Build history of the part. All positions in model axes, mm. A direction names the side the tool comes from. Round coordinates to 2 decimals unless told otherwise and drop trailing zeros. Write each loop counter-clockwise with the first axis right and the second up, starting at its lowest first coordinate (ties: lowest second). Pieces come first, ordered by that corner, then holes. Notation, with made-up numbers: M 52.25,-2 L 91.25,-2 A29 cw 91.25,21 Z; hole C -25.75,45 d5. An arc over 180 degrees is marked long. One line per item, written item: value. Start each with the question number.
```python
from build123d import *

# Parameters (mm, degrees)
SKETCH1_R               = 40
SKETCH1_R_2             = 7.5
BOSS_EXTRUDE1_DEPTH     = 7.5
CUT_EXTRUDE1_REACH      = 59.064
CUT_EXTRUDE1_END_RADIUS = 40
SKETCH2_R               = 2
CUT_EXTRUDE2_REACH      = 99.064
CUT_EXTRUDE2_END_RADIUS = 7.5
CUT_EXTRUDE2_START      = 40
SKETCH2_2_R             = 2


with BuildPart() as part:
    # Sketch1 → Boss-Extrude1 (new, symmetric)
    with BuildSketch(Plane.XY):
        Circle(SKETCH1_R)
        with Locations((26, 0)):
            Circle(SKETCH1_R_2, mode=Mode.SUBTRACT)
        with BuildLine():
            Line((4.769696007, 1.5), (6.5, 1.5))
            Line((6.5, 1.5), (6.5, -1.5))
            Line((6.5, -1.5), (4.769696007, -1.5))
            ThreePointArc((4.769696007, -1.5), (-5, 0), (4.769696007, 1.5))
        make_face(mode=Mode.SUBTRACT)
    extrude(amount=BOSS_EXTRUDE1_DEPTH, both=True)

    # Cut-Extrude1: up to this cylinder (the profile starts inside it)
    cut_extrude1_end = Plane(origin=(0, 0, 0), z_dir=(0, 0, -1)) * Cylinder(CUT_EXTRUDE1_END_RADIUS, 199.128, mode=Mode.PRIVATE)
    # Sketch2 → Cut-Extrude1 (cut, up to the surface)
    with BuildSketch(Plane(origin=(0, 0, 0), x_dir=(0, 0, -1), z_dir=(1, 0, 0)), mode=Mode.PRIVATE) as cut_extrude1_sk1:
        Circle(SKETCH2_R)
    cut_extrude1_tool1 = extrude(cut_extrude1_sk1.sketch, amount=-CUT_EXTRUDE1_REACH, mode=Mode.PRIVATE) & cut_extrude1_end
    add(cut_extrude1_tool1.solids().sort_by_distance((0, 0, 0))[0], mode=Mode.SUBTRACT)

    # Cut-Extrude2: up to this cylinder (the profile starts outside it)
    cut_extrude2_end = Plane(origin=(26, 0, 0), z_dir=(0, 0, -1)) * Cylinder(CUT_EXTRUDE2_END_RADIUS, 214.128, mode=Mode.PRIVATE)
    # Sketch2<2> → Cut-Extrude2 (cut, up to the surface)
    with BuildSketch(Plane(origin=(0, 0, 0), x_dir=(0, 0, -1), z_dir=(1, 0, 0)).offset(CUT_EXTRUDE2_START), mode=Mode.PRIVATE) as cut_extrude2_sk1:
        Circle(SKETCH2_2_R)
    cut_extrude2_tool1 = extrude(cut_extrude2_sk1.sketch, amount=-CUT_EXTRUDE2_REACH, mode=Mode.PRIVATE) - cut_extrude2_end
    add(cut_extrude2_tool1.solids().sort_by_distance((40, 0, 0))[0], mode=Mode.SUBTRACT)


solid = part.part
```
Item 1: Which spindle directions (+Z, -Z, +X, -X, +Y, -Y) get a long thin tool onto all of the face, cutting with end or side? Do faces 1 (the flat face through (-1, -8, 7.5)), 2 (the flat face through (6.5, 0, 0)), 3 (the cylindrical face through (37, -2, 0)). Say none if no direction does.
Item 2: Two-plate mould, pull along X, no slides. Class faces 4 (the cylindrical face through (-22, -2, 0)), 5 (the flat face through (6, -1.5, 0)), 6 (the cylindrical face through (38.153, 12.015, 0.105)), 7 (the cylindrical face through (18.507, 0.33, -0.105)): pulls with the +X half, pulls with the -X half, needs draft (parallel to the pull), parting line crosses it, or undercut.
Item 3: Cut at D-D, the plane z = 0. Write the cut outline in (x, y).
Item 4: Cut at C-C, the plane z = -5. Write the cut outline in (x, y).
Item 5: Drill centre lines: line 1 (Y direction, x = 0, z = 3); line 2 (Z direction, x = 38.5, y = 0); line 3 (Y direction, x = -34, z = 1.25). Where is each one in solid material? Low to high.
Item 6: Cut at B-B, the plane y = 0. Write the cut outline in (x, z), plus the area to 4 significant figures.
Item 7: Drop flat-ended pins along their axis: pin 1 (5 mm diameter, centred on y = -20.5, z = -1, fed in from -X); pin 2 (3 mm diameter, centred on x = 8.5, z = 5.5, fed in from +Y); pin 3 (3 mm diameter, centred on y = 0, z = 0, fed in from +X); pin 4 (24 mm diameter, centred on x = 26, y = 0, fed in from -Z). Give the stop position or say it passes through.
Item 8: Cut at A-A, the plane x = 0. Write the cut outline in (y, z), plus the area to 3 significant figures.
Computed values:
1. face 1: +Z, +X, -X, +Y, -Y
1. face 2: +Z, -Z
1. face 3: +X
2. face 4: needs draft
2. face 5: undercut
2. face 6: parting line crosses it
2. face 7: undercut
3. outline: M -39.95,-2 A40 ccw 39.95,-2 L 33.23,-2 A7.5 cw long 33.23,2 L 39.95,2 A40 ccw -39.95,2 L -4.58,2 A5 cw 4.77,1.5 L 6.5,1.5 L 6.5,-1.5 L 4.77,-1.5 A5 cw -4.58,-2 Z
4. outline: C 0,0 d80; hole M 4.77,-1.5 L 6.5,-1.5 L 6.5,1.5 L 4.77,1.5 A5 ccw long Z; hole C 26,0 d15
5. line 1: y = -40 to -5, 5 to 40
5. line 2: z = -7.5 to -2, 2 to 7.5
5. line 3: y = -21.07 to -1.56, 1.56 to 21.07
6. outline: M -40,-7.5 L -5,-7.5 L -5,-2 L -40,-2 Z; M -40,2 L -5,2 L -5,7.5 L -40,7.5 Z; M 6.5,-7.5 L 18.5,-7.5 L 18.5,7.5 L 6.5,7.5 Z; M 33.5,-7.5 L 40,-7.5 L 40,-2 L 33.5,-2 Z; M 33.5,2 L 40,2 L 40,7.5 L 33.5,7.5 Z
6. area: 636.5 mm2
7. pin 1: stops at x = -35.72
7. pin 2: stops at y = 39.38
7. pin 3: stops at x = 18.65
7. pin 4: stops at z = -7.5
8. outline: M -40,-7.5 L -5,-7.5 L -5,7.5 L -40,7.5 Z; M 5,-7.5 L 40,-7.5 L 40,7.5 L 5,7.5 Z
8. area: 1,050 mm2
